```python
from build123d import *

# Parameters (mm, degrees)
F0_R     = 22.225
F0_R_2   = 12.827
F0_R_3   = 3.9414525169
F1_DEPTH = 76.2
F2_DEPTH = 58.42
F3_START = 71.628
F3_DEPTH = 385.572


with BuildPart() as f1:
    # F0 (on Top) → F1 (new body)
    with BuildSketch(Plane.XY):
        Circle(F0_R)
        Circle(F0_R_2, mode=Mode.SUBTRACT)
        Circle(F0_R_2)
        Circle(F0_R_3, mode=Mode.SUBTRACT)
        Circle(F0_R_3)
    extrude(amount=F1_DEPTH)

    # F0 (on Top) → F2 (cut)
    with BuildSketch(Plane.XY):
        Circle(F0_R_2)
        Circle(F0_R_3, mode=Mode.SUBTRACT)
        Circle(F0_R_3)
    extrude(amount=F2_DEPTH, mode=Mode.SUBTRACT)

    # F0 (on Top) → F3 (join)
    with BuildSketch(Plane.XY.offset(F3_START)):
        Circle(F0_R_2)
        Circle(F0_R_3, mode=Mode.SUBTRACT)
    extrude(amount=F3_DEPTH)


solid = f1.part
```
The model under review builds one solid part; all positions refer to its coordinate system, in mm. A direction names the side the tool comes from. Round coordinates to 2 decimals unless told otherwise and drop trailing zeros. Order: outer loops, then holes, each group sorted by start corner. A loop starts at its lowest first (then second) coordinate and runs counter-clockwise, first axis right, second up.
Item 1: For pin 1 (1.5 mm diameter, centred on x = -11, z = 214, fed in from +Y); pin 2 (6 mm diameter, centred on x = 4.5, z = 229, fed in from +Y); pin 3 (5 mm diameter, centred on x = 6.5, y = -14, fed in from +Z); pin 4 (8 mm diameter, centred on y = 2, z = 71.5, fed in from -X) (3 decimals), all flat-tipped, find the tip position at first contact; note any pin that passes through.
Working result:
pin 1: stops at y = 7.71
pin 2: stops at y = 12.74
pin 3: stops at z = 76.2
pin 4: stops at x = -22.225
Item 2: Add section D-D, the plane z = 43. State the section outline as (x, y) points (3 decimals).
Working result:
outline: circle Ø44.45 at (0, 0); hole circle Ø25.654 at (0, 0)
Item 3: Add section C-C, the plane z = 294. State the section outline as (x, y) points.
Working result:
outline: circle Ø25.65 at (0, 0); hole circle Ø7.88 at (0, 0)
Item 4: Draft analysis for pull direction X (two halves, no side actions). For faces 1 (the flat face through (10, -10, 76.2)), 2 (the cylindrical face through (12.235, 3.853, 28.801)), 3 (the cylindrical face through (21.199, 6.676, 37.567)), state which applies: released by +X, released by -X, zero draft, split by the parting line, or undercut.
Working result:
face 1: zero draft
face 2: undercut
face 3: split by the parting line
Item 5: Machinability: for faces 4 (the flat face through (10, -10, 0)), 5 (the cylindrical face through (12.235, 3.853, 264.033)), 6 (the flat face through (0, 0, 58.42)), which of the approach directions +Z, -Z, +X, -X, +Y, -Y give a long, thin tool a straight path to every point of the face, cutting with its end or side? Answer none if there is none.
Working result:
face 4: -Z, +X, -X, +Y, -Y
face 5: +Z
face 6: -Z
Item 6: Add section A-A, the plane y = 0. State the section outline as (x, z) points (3 decimals), and give its area (3 significant figures).
Working result:
outline: (-22.225, 0) - (-12.827, 0) - (-12.827, 58.42) - (12.827, 58.42) - (12.827, 0) - (22.225, 0) - (22.225, 76.2) - (12.827, 76.2) - (12.827, 457.2) - (3.941, 457.2) - (3.941, 76.2) - (-3.941, 76.2) - (-3.941, 457.2) - (-12.827, 457.2) - (-12.827, 76.2) - (-22.225, 76.2) - close
area: 8,660 mm2
Item 7: To check wall thickness, follow probe 1 along X at (y, z) = (0, 290); probe 2 along Z at (x, y) = (-1, -1); probe 3 along Y at (x, z) = (0, 20) (3 decimals). State the ranges of each line that lie inside material, in increasing order.
Working result:
probe 1: x = -12.83 to -3.94, 3.94 to 12.83
probe 2: z = 58.42 to 76.2
probe 3: y = -22.225 to -12.827, 12.827 to 22.225
